```python
from build123d import *

# Parameters (mm, degrees)
SKETCH1_W               = 76.2
SKETCH1_H               = 50.8
BOSS_EXTRUDE1_DEPTH     = 12.7
SKETCH2_R               = 3.175
CUT_EXTRUDE1_DEPTH      = 65.757547823
SKETCH3_R               = 4.7625
CUT_EXTRUDE2_DEPTH      = 65.757547823
F_1_4_CLEARANCE_HOLE1_D = 6.7564
F_8_CLEARANCE_HOLE1_D   = 4.4958
SKETCH8_R               = 6.096
CUT_EXTRUDE3_DEPTH      = 3.175


with BuildPart() as part:
    # Sketch1 → Boss-Extrude1 (new body)
    with BuildSketch(Plane(origin=(0, 0, 0), x_dir=(1, 0, 0), z_dir=(0, 1, 0))):
        Rectangle(SKETCH1_W, SKETCH1_H)
    extrude(amount=BOSS_EXTRUDE1_DEPTH)

    # Sketch2 → Cut-Extrude1 (cut, through all)
    with BuildSketch(Plane.XY.offset(25.4)):
        with Locations((-25.4, 12.7)):
            Circle(SKETCH2_R)
        with Locations((25.4, 12.7)):
            Circle(SKETCH2_R)
    extrude(amount=-CUT_EXTRUDE1_DEPTH, mode=Mode.SUBTRACT)

    # Sketch3 → Cut-Extrude2 (cut, through all)
    with BuildSketch(Plane.XY.offset(25.4)):
        with Locations((-9.525, 12.7)):
            Circle(SKETCH3_R)
        with Locations((9.525, 12.7)):
            Circle(SKETCH3_R)
    extrude(amount=-CUT_EXTRUDE2_DEPTH, mode=Mode.SUBTRACT)

    # 1/4 Clearance Hole1 (through all)
    with Locations(Plane(origin=(0, 12.7, 0), x_dir=(1, 0, 0), z_dir=(0, 1, 0))):
        with Locations((-33.3375, -19.05), (-33.3375, 19.05), (33.3375, 19.05), (33.3375, -19.05)):
            Hole(F_1_4_CLEARANCE_HOLE1_D / 2)

    # #8 Clearance Hole1 (through all)
    with Locations(Plane(origin=(0, 12.7, 0), x_dir=(1, 0, 0), z_dir=(0, 1, 0))):
        with Locations((-19.05, -19.05), (-19.05, 19.05), (0, 12.7), (0, -12.7), (19.05, -19.05), (19.05, 19.05)):
            Hole(F_8_CLEARANCE_HOLE1_D / 2)

    # Sketch8 → Cut-Extrude3 (cut)
    with BuildSketch(Plane.XZ):
        with Locations(Location((-19.05, 19.05, 0), (0, 0, 270))):
            Circle(SKETCH8_R)
        with Locations(Location((0, 12.7, 0), (0, 0, 270))):
            Circle(SKETCH8_R)
        with Locations(Location((19.05, 19.05, 0), (0, 0, 270))):
            Circle(SKETCH8_R)
        with Locations(Location((19.05, -19.05, 0), (0, 0, 270))):
            Circle(SKETCH8_R)
        with Locations(Location((-19.05, -19.05, 0), (0, 0, 270))):
            Circle(SKETCH8_R)
        with Locations(Location((0, -12.7, 0), (0, 0, 270))):
            Circle(SKETCH8_R)
    extrude(amount=-CUT_EXTRUDE3_DEPTH, mode=Mode.SUBTRACT)


solid = part.part
```
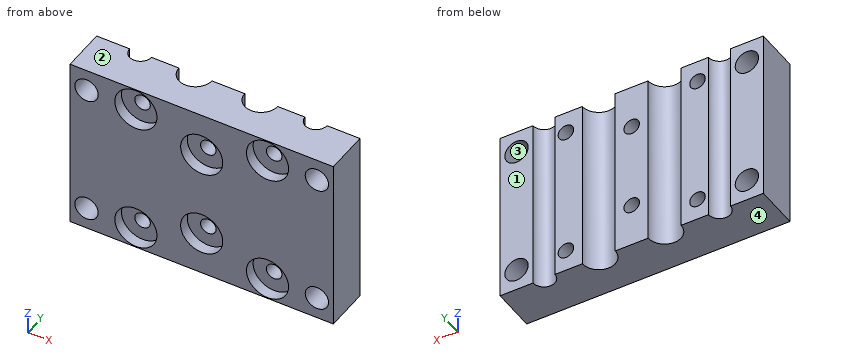
Model file for the job. Use its own axes, mm. Face numbers are marked on the shaded views. Round coordinates to 2 decimals unless told otherwise and drop trailing zeros. Write each loop counter-clockwise with the first axis right and the second up, starting at its lowest first coordinate (ties: lowest second). Pieces come first, ordered by that corner, then holes. Notation, with made-up numbers: (28, 60) - (80, 60) arc R23 cw to (80, 81) - close; hole circle Ø2 at (33, 17). An arc over 180 degrees is marked (long way). One line per item, written item: value.
(1) Cut at A-A, the plane x = 0. Give the cut face in (y, z) (3 decimals).
Values follow:
outline: (0, -25.4) - (12.7, -25.4) - (12.7, -14.948) - (3.175, -14.948) - (3.175, -18.796) - (0, -18.796) - close; (0, -6.604) - (3.175, -6.604) - (3.175, -10.452) - (12.7, -10.452) - (12.7, 10.452) - (3.175, 10.452) - (3.175, 6.604) - (0, 6.604) - close; (0, 18.796) - (3.175, 18.796) - (3.175, 14.948) - (12.7, 14.948) - (12.7, 25.4) - (0, 25.4) - close
(2) Drop flat-ended pins along their axis: P1, Ø11, axis at x = 0, z = -12.7, coming from the -Y side (3 decimals); P2, Ø10, axis at x = -0.5, z = -15, coming from the -Y side. Give the stop position or say it passes through.
Values follow:
P1: stops at y = 3.175
P2: stops at y = 0
(3) Two-plate mould, pull along Z, no slides. Class the marked faces 1, 2, 3 and 4: pulls with the +Z half, pulls with the -Z half, needs draft (parallel to the pull), parting line crosses it, or undercut.
Values follow:
face 1: needs draft
face 2: pulls with the +Z half
face 3: undercut
face 4: pulls with the -Z half
(4) Wall check: probe 1 along X at (y, z) = (1.55, 19.05); probe 2 along Z at (x, y) = (19.05, 5.75); probe 3 along X at (y, z) = (11.5, -15.5). Give the ranges that are in metal, low to high.
Values follow:
probe 1: x = -38.1 to -36.72, -29.96 to -25.15, -12.95 to 12.95, 25.15 to 29.96, 36.72 to 38.1
probe 2: z = -25.4 to -21.3, -16.8 to 16.8, 21.3 to 25.4
probe 3: x = -38.1 to -28.34, -22.46 to -14.13, -4.92 to 4.92, 14.13 to 22.46, 28.34 to 38.1
(5) Cut at B-B, the plane y = 11.75. Give the number of separate pieces and of enclosed holes in the cut face, plus the area to 3 significant figures.
Values follow:
separate pieces: 5
enclosed holes: 10
area: 2,070 mm²
